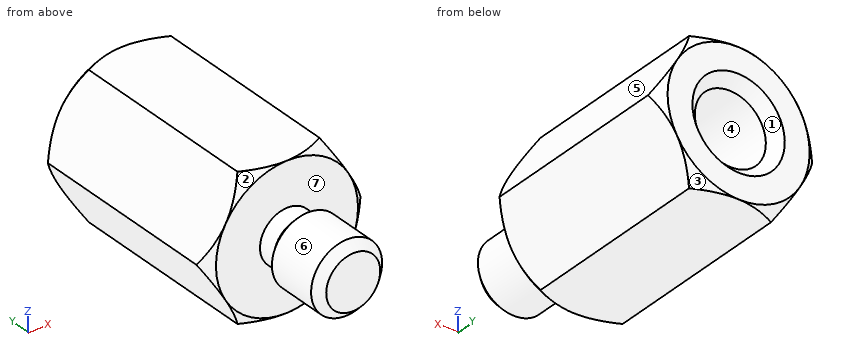
```python
from build123d import *

# Parameters (mm, degrees)
EXTRUDE1_DEPTH = 6


with BuildPart() as part:
    # Sketch1 → Extrude1 (new body)
    with BuildSketch(Plane(origin=(0, 0, 0), x_dir=(1, 0, 0), z_dir=(0, 1, 0))):
        Polygon((1.154700538, 2), (-1.154700538, 2), (-2.309401077, 0), (-1.154700538, -2), (1.154700538, -2), (2.309401077, 0), align=None)
    extrude(amount=EXTRUDE1_DEPTH)

    # Sketch2 → Revolve1 (revolve)
    with BuildSketch(Plane(origin=(0, 0, 0), x_dir=(0, 0, -1), z_dir=(1, 0, 0)), mode=Mode.PRIVATE) as revolve1_sk:
        Polygon((0.76, 0), (0.76, -0.5), (1, -0.74), (1, -2.16), (0.76, -2.4), (0, -2.4), (0, 0), align=None)
    revolve(revolve1_sk.sketch.rotate(Axis((0, 0, 0), (0, -1, 0)), 180), axis=Axis((0, 0, 0), (0, -1, 0)))

    # Sketch3 → Cut-Revolve1 (revolve, cut)
    with BuildSketch(Plane(origin=(0, 0, 0), x_dir=(0, 0, -1), z_dir=(1, 0, 0)), mode=Mode.PRIVATE) as cut_revolve1_sk:
        Polygon((1.3, 6), (1, 5.7), (1, 2.4), (0, 1.799139381), (0, 6), align=None)
    revolve(cut_revolve1_sk.sketch.rotate(Axis((0, 6, 0), (0, -1, 0)), 180), axis=Axis((0, 6, 0), (0, -1, 0)), mode=Mode.SUBTRACT)

    # Sketch4 → Cut-Revolve3 (revolve, cut)
    with BuildSketch(Plane(origin=(0, 0, 0), x_dir=(0, 0, -1), z_dir=(1, 0, 0))):
        Polygon((2, 6), (4.5, 6), (4.5, 3.5), align=None)
        Polygon((2, 0), (4.5, 0), (4.5, 2.5), align=None)
    revolve(axis=Axis((0, 0, 0), (0, 1, 0)), mode=Mode.SUBTRACT)


solid = part.part
```
Work out the finished part from the listing and answer in its coordinate system (mm). Face numbers are marked on the shaded views. A direction names the side the tool comes from. Round coordinates to 2 decimals unless told otherwise and drop trailing zeros. Write each loop counter-clockwise with the first axis right and the second up, starting at its lowest first coordinate (ties: lowest second). Pieces come first, ordered by that corner, then holes. Notation, with made-up numbers: (-25, -16.75) - (9, -16.75) arc R16 ccw to (9, -3.75) - close; hole circle Ø11 at (87, 64.5). An arc over 180 degrees is marked (long way). Return JSON: item names as keys, results as strings. Group by question number.
Q1. This flat-tipped pin is pushed along its axis until it touches: pin 1 Ø1.5 at (x, z) = (-1.5, 1) entering from -Y. Where does it stop, or does it pass through?
Q2. The mould has two halves that part along Z. Classify the marked faces 1, 2, 3 and 4: released by +Z, released by -Z, zero draft, split by the parting line, or undercut.
Q3. The part is cut by section A-A on y = 4. Write down the section's boundary in (x, z).
Q4. Find the intervals of material crossed by L1, parallel to Y at x = 0.6, z = 1.7; L2, parallel to X at y = 3.5, z = 0.6; L3, parallel to X at y = 5.5, z = 0.45, in increasing order.
Q5. For the marked faces 5, 6 and 7, determine the directions among +Z, -Z, +X, -X, +Y, -Y from which every point of the face is accessible in a straight line to the end or side of a thin tool.
Solved:
{
 "1": {"pin 1": "y = 0"},
 "2": {"face 1": "undercut", "face 2": "released by +Z", "face 3": "released by -Z", "face 4": "undercut"},
 "3": {"outline": "(-2.31, 0) - (-1.15, -2) - (1.15, -2) - (2.31, 0) - (1.15, 2) - (-1.15, 2) - close; hole circle Ø2 at (0, 0)"},
 "4": {"L1": "0 to 6", "L2": "-1.96 to -0.8, 0.8 to 1.96", "L3": "-2.05 to -0.89, 0.89 to 2.05"},
 "5": {"face 5": "+Z, +X, +Y, -Y", "face 6": "-Y", "face 7": "none"}
}
